Design review of the part built by this model. Coordinates are the model's own, in mm. Face numbers are marked on the shaded views. A direction names the side the tool comes from. Coordinates: 2 decimals unless noted, no trailing zeros. Loops run counter-clockwise (first coordinate to the right, second up) from the corner with the lowest first, then second, coordinate; pieces in that order, holes last. Notation, with made-up numbers: (33, 72.5) -> (76, 72.5) arc R28 cw to (76, 93.5) -> close; hole circle Ø9 at (51, 50.25). An arc over 180 degrees is marked (long way). Use a Markdown table: item, result. Add a question column.
Q1. Take a section at D-D on x = 10.5. Write out the cut boundary in (y, z) (3 decimals).
Q2. Draft analysis for pull direction Z (two halves, no side actions). For the marked faces 1, 2 and 3, state which applies: pulls with the +Z half, pulls with the -Z half, needs draft (parallel to the pull), parting line crosses it, or undercut.
Q3. For the marked faces 4, 5, 6, 7 and 8, list the 3-axis set-ups (+Z, -Z, +X, -X, +Y, -Y) from which the entire face can be reached by the end or side of a thin tool; tool diameter is ignored.
Q4. Clearance check with flat-ended pins moving along their axes: pin 1 Ø4 at (y, z) = (-14, 6.5) entering from +X; pin 2 Ø1.5 at (x, z) = (-22, 0) entering from -Y; pin 3 Ø5.5 at (x, z) = (10, -1.75) entering from -Y; pin 4 Ø4 at (x, y) = (13.5, -17.5) entering from -Z. State where each tip first meets the part, or that it passes through.
Q5. Take a section at A-A on y = 0. Write out the cut boundary in (x, z), plus the area to 3 significant figures.
Q6. Take a section at C-C on y = -14. Write out the cut boundary in (x, z), plus the area to 3 significant figures.
Q7. Take a section at B-B on x = -10. Write out the cut boundary in (y, z) (3 decimals).
Q8. For probe 1 along X at (y, z) = (-21, 10.5); probe 2 along X at (y, z) = (17.5, 8.5); probe 3 along X at (y, z) = (-3, 7.75), list the stretches that pass through material, from the lowest coordinate up.
Solid Edge part; units mm, degrees
sketch "Sketch1" plane through (0, 0, 0) normal (0, 0, 1) x (1, 0, 0)
  line L0 (23.5, -23.5) -> (20.5, -23.5)
  line L1 (20.5, 17) -> (20.5, -23.5)
  line L2 (-20.5, 17) -> (20.5, 17)
  line L3 (-20.5, -23.5) -> (-20.5, 17)
  line L4 (-20.5, -23.5) -> (-23.5, -23.5)
  line L5 (-23.5, -23.5) -> (-23.5, 23.5)
  line L6 (-23.5, 23.5) -> (23.5, 23.5)
  line L7 (23.5, 23.5) -> (23.5, -23.5)
  dimension "D1" = 20.5
  dimension "D2" = 20.5
  dimension "D3" = 23.5
  dimension "D4" = 20.5
  dimension "D5" = 23.5
extrude "ProtrusiónExtruida_1" add sketch "Sketch1" along normal mid plane 16
sketch "Sketch2" plane through (0, 0, 8) normal (0, 0, 1) x (1, 0, 0)
  line L0 (23.5, -23.5) -> (-23.5, -23.5)
  line L1 (-23.5, -23.5) -> (-23.5, 23.5)
  line L2 (-23.5, 23.5) -> (23.5, 23.5)
  line L3 (23.5, 23.5) -> (23.5, -23.5)
extrude "Protrusion1" add sketch "Sketch2" along normal blind 4
sketch "Sketch3" plane through (-23.5, 0, -2.5) normal (-1, 0, 0) x (0, 1, 0)
  line L0 (14, -4.5) -> (9, -4.5)
  line L1 (14, 0.5) -> (14, -4.5)
  dimension "D1" = 14
extrude "Cutout1" cut sketch "Sketch3" against normal through all material side at (-23.5, 11.5, 1.95)
sketch "Sketch4" plane through (0, 17, 0) normal (0, -1, 0) x (-1, 0, 0)
  line L0 (8.3401, 4.625) -> (11.6599, 4.625)
  line L1 (11.6599, 4.625) -> (13.3198, 1.75)
  line L2 (13.3198, 1.75) -> (11.6599, -1.125)
  line L3 (11.6599, -1.125) -> (8.3401, -1.125)
  line L4 (8.3401, -1.125) -> (6.6802, 1.75)
  line L5 (6.6802, 1.75) -> (8.3401, 4.625)
extrude "VaciadoExtruido_18" cut sketch "Sketch4" against normal blind 5
sketch "Sketch5" plane through (0, 23.5, -2.5) normal (0, 1, 0) x (1, 0, 0)
  circle A0 centre (-10, -0.75) radius 1.65
  dimension "D1" = 10
extrude "Cutout2" cut sketch "Sketch5" against normal up to next
chamfer "Chaflán_1" distance 10 angle 45 2 edges at (-23.5, 18.75, -8) (23.5, 18.75, -8)
fillet "Redondeo_5" radius 10 2 edges at (-13.5, 20.25, -8) (13.5, 20.25, -8)
sketch "Sketch6" plane through (0, -4.5, 8) normal (0, 0, -1) x (-1, 0, 0)
  line L0 (-22.7321, -13.5) -> (-19.2679, -13.5)
  line L1 (-19.2679, -13.5) -> (-17.5359, -16.5)
  line L2 (-17.5359, -16.5) -> (-19.2679, -19.5)
  line L3 (-19.2679, -19.5) -> (-22.7321, -19.5)
  line L4 (-24.8409, -19.8273) -> (-22.7321, -19.5)
  line L5 (-24.4641, -16.5) -> (-24.8409, -19.8273)
  line L6 (-24.4641, -16.5) -> (-22.7321, -13.5)
  line L7 (19.2679, -13.5) -> (22.7321, -13.5)
  line L8 (22.7321, -13.5) -> (24.4641, -16.5)
  line L9 (25.4467, -19.5) -> (24.4641, -16.5)
  line L10 (22.7321, -19.5) -> (25.4467, -19.5)
  line L11 (22.7321, -19.5) -> (19.2679, -19.5)
  line L12 (19.2679, -19.5) -> (17.5359, -16.5)
  line L13 (17.5359, -16.5) -> (19.2679, -13.5)
  line L14 (19.2679, 28.5) -> (22.7321, 28.5)
  line L15 (22.7321, 28.5) -> (25.2223, 28.8412)
  line L16 (25.2223, 28.8412) -> (24.4641, 25.5)
  line L17 (24.4641, 25.5) -> (22.7321, 22.5)
  line L18 (22.7321, 22.5) -> (19.2679, 22.5)
  line L19 (19.2679, 22.5) -> (17.5359, 25.5)
  line L20 (17.5359, 25.5) -> (15.8038, 28.5)
  line L21 (15.8038, 28.5) -> (19.2679, 28.5)
  line L22 (-22.7321, 28.5) -> (-19.2679, 28.5)
  line L23 (-19.2679, 28.5) -> (-15.8038, 28.5)
  line L24 (-15.8038, 28.5) -> (-17.5359, 25.5)
  line L25 (-17.5359, 25.5) -> (-19.2679, 22.5)
  line L26 (-19.2679, 22.5) -> (-22.7321, 22.5)
  line L27 (-22.7321, 22.5) -> (-24.4641, 25.5)
  line L28 (-25.1936, 28.5) -> (-24.4641, 25.5)
  line L29 (-22.7321, 28.5) -> (-25.1936, 28.5)
extrude "VaciadoExtruido_32" cut sketch "Sketch6" against normal blind 1 and the other way up to next
sketch "Sketch7" plane through (9, -9, 12) normal (0, 0, 1) x (0, -1, 0)
  circle A0 centre (-30, -30) radius 1.65
  circle A1 centre (12, -30) radius 1.65
  circle A2 centre (12, 12) radius 1.65
  circle A3 centre (-30, 12) radius 1.65
extrude "Cutout3" cut sketch "Sketch7" against normal up to next
sketch "Sketch8" plane through (0, -4.5, 8) normal (0, 0, -1) x (-1, 0, 0)
  line L0 (-2.75, -19) -> (2.75, -19)
  line L1 (2.75, -19) -> (2.75, -20.75)
  line L2 (2.75, -20.75) -> (-2.75, -20.75)
  line L3 (-2.75, -20.75) -> (-2.75, -19)
  dimension "D1" = 2.75
  dimension "D2" = 2.75
revolve "VaciadoPorRevolución_1" cut sketch "Sketch8" angle 90 about axis through (4.4935, -21.7, 8) along (-1, 0, 0)
sketch "Sketch9" plane through (0, -21.7, 11.25) normal (0, -1, 0) x (-1, 0, 0)
  line L0 (-2.75, 1.45) -> (2.75, 1.45)
  line L1 (2.75, 1.45) -> (2.75, -0.3)
  line L2 (2.75, -0.3) -> (-2.75, -0.3)
  line L3 (-2.75, -0.3) -> (-2.75, 1.45)
extrude "VaciadoExtruido_34" cut sketch "Sketch9" against normal blind 34
sketch "Sketch10" plane through (0, 12.3, 11.25) normal (0, -1, 0) x (-1, 0, 0)
  line L0 (-2.75, -0.3) -> (-2.75, 1.45)
  line L1 (-2.75, 1.45) -> (2.75, 1.45)
  line L2 (2.75, 1.45) -> (2.75, -0.3)
  line L3 (2.75, -0.3) -> (-2.75, -0.3)
revolve "RevolvedCutout1" cut sketch "Sketch10" angle 90 about axis through (2.8162, 12.3, 2.8) along (-1, 0, 0)
sketch "Sketch11" plane through (0, 18.25, 2.8) normal (0, 0, 1) x (1, 0, 0)
  line L0 (2.75, 1.05) -> (-2.75, 1.05)
  line L1 (-2.75, 1.05) -> (-2.75, 2.8)
  line L2 (-2.75, 2.8) -> (2.75, 2.8)
  line L3 (2.75, 2.8) -> (2.75, 1.05)
extrude "Cutout4" cut sketch "Sketch11" against normal up to next
fillet "Redondeo_6" radius 2 1 edges at (0, 19.3, -8)
sketch "Sketch12" plane through (22, -2, -8) normal (0, 0, -1) x (0, -1, 0)
  line L0 (-4.75, 0.25) -> (0.75, 0.25)
  line L1 (0.75, 0.25) -> (0.75, -1.5)
  line L2 (0.75, -1.5) -> (-4.75, -1.5)
  line L3 (-4.75, -1.5) -> (-4.75, 0.25)
  dimension "D1" = 4.75
  dimension "D2" = 0.75
extrude "Cutout5" cut sketch "Sketch12" against normal up to surface (16 mm away)
sketch "Sketch13" plane through (22.75, 0, 8) normal (0, 0, -1) x (-1, 0, 0)
  line L0 (1, 2.75) -> (-0.75, 2.75)
  line L1 (-0.75, 2.75) -> (-0.75, -2.75)
  line L2 (-0.75, -2.75) -> (1, -2.75)
  line L3 (1, -2.75) -> (1, 2.75)
revolve "VaciadoPorRevolución_3" cut sketch "Sketch13" angle 90 about axis through (20.25, 2.6731, 8) along (0, -1, 0)
sketch "Sketch14" plane through (20.25, 0, 11.25) normal (1, 0, 0) x (0, -1, 0)
  line L0 (-2.75, 1.75) -> (-2.75, 0)
  line L1 (-2.75, 0) -> (2.75, 0)
  line L2 (2.75, 0) -> (2.75, 1.75)
  line L3 (2.75, 1.75) -> (-2.75, 1.75)
extrude "VaciadoExtruido_37" cut sketch "Sketch14" against normal blind 33
mirror "Mirror1" about plane through (0, 0, 0) normal (1, 0, 0) of "Cutout2", "VaciadoExtruido_18", "Cutout5", "VaciadoPorRevolución_3", "VaciadoExtruido_37"
sketch "Sketch15" plane through (0, -4.5, 8) normal (0, 0, -1) x (0, -1, 0)
  line L0 (5, 27.5098) -> (5, -27.4354)
extrude "Cutout10" cut sketch "Sketch15" along normal through all material side at (-0.0372, -9.55, 8)
sketch "Sketch16" plane through (0, -4, 11.25) normal (0, 0, -1) x (-1, 0, 0)
  line L0 (-2.75, 1.25) -> (-2.75, -2.5)
  line L1 (-2.75, -2.5) -> (2.75, -2.5)
  line L2 (2.75, 1.25) -> (2.75, -2.5)
  line L3 (6.5, 1.25) -> (2.75, 1.25)
  line L4 (6.5, 1.25) -> (6.5, 6.75)
  line L5 (6.5, 6.75) -> (2.75, 6.75)
  line L6 (2.75, 10.5) -> (2.75, 6.75)
  line L7 (2.75, 10.5) -> (-2.75, 10.5)
  line L8 (-2.75, 10.5) -> (-2.75, 6.75)
  line L9 (-2.75, 6.75) -> (-6.5, 6.75)
  line L10 (-6.5, 6.75) -> (-6.5, 1.25)
  line L11 (-2.75, 1.25) -> (-6.5, 1.25)
extrude "Cutout11" cut sketch "Sketch16" against normal up to next
sketch "Sketch17" plane through (0, -3.25, 8) normal (0, 0, -1) x (1, 0, 0)
  line L0 (-2.75, 16.75) -> (2.75, 16.75)
  line L1 (2.75, 16.75) -> (2.75, 20.25)
  line L2 (2.75, 20.25) -> (-2.75, 20.25)
  line L3 (-2.75, 16.75) -> (-2.75, 20.25)
extrude "Cutout12" cut sketch "Sketch17" against normal up to next
properties material "Abs 15"
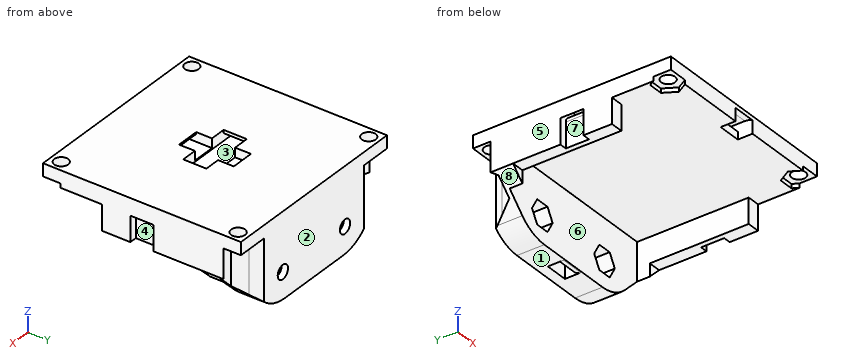
Answer list:
| question | item | result |
|---|---|---|
| 1 | outline | (-23.5, 8) -> (17, 8) -> (17, 1.125) -> (22, 1.125) -> (22, -0.178) -> (23.5, -0.178) -> (23.5, 12) -> (-23.5, 12) -> close; (17, -7.935) -> (23.5, -7.935) -> (23.5, -3.322) -> (22, -3.322) -> (22, -4.625) -> (17, -4.625) -> close; hole (-2.75, 9.5) -> (2.75, 9.5) -> (2.75, 11.25) -> (-2.75, 11.25) -> close |
| 2 | face 1 | pulls with the -Z half |
| 2 | face 2 | needs draft |
| 2 | face 3 | undercut |
| 3 | face 4 | -Z, +X |
| 3 | face 5 | +Z, -Z, -X, +Y, -Y |
| 3 | face 6 | -Z, -Y |
| 3 | face 7 | -Z, -X |
| 3 | face 8 | -Z, -X, +Y, -Y |
| 4 | pin 1 | x = 23.5 |
| 4 | pin 2 | y = 14 |
| 4 | pin 3 | y = 22 |
| 4 | pin 4 | z = 8 |
| 5 | outline | (-23.5, 8) arc R3.25 cw to (-20.25, 11.25) -> (-6.5, 11.25) -> (-6.5, 12) -> (-23.5, 12) -> close; (-21.75, 2) -> (-20.5, 2) -> (-20.5, 8) -> (20.5, 8) -> (20.5, 2) -> (21.75, 2) -> (21.75, 8) arc R1.5 ccw to (20.25, 9.5) -> (-20.25, 9.5) arc R1.5 ccw to (-21.75, 8) -> close; (6.5, 11.25) -> (20.25, 11.25) arc R3.25 cw to (23.5, 8) -> (23.5, 12) -> (6.5, 12) -> close |
| 5 | area | 109 mm² |
| 6 | outline | (-23.5, 8) -> (23.5, 8) -> (23.5, 12) -> (-23.5, 12) -> close; hole (-2.75, 9.8) -> (2.75, 9.8) -> (2.75, 11.55) -> (-2.75, 11.55) -> close |
| 6 | area | 178 mm² |
| 7 | outline | (-23.5, 8) -> (17, 8) -> (17, 1.125) -> (22, 1.125) -> (22, -0.1) -> (23.5, -0.1) -> (23.5, 12) -> (-23.5, 12) -> close; (17, -7.979) -> (23.5, -7.979) -> (23.5, -3.4) -> (22, -3.4) -> (22, -4.625) -> (17, -4.625) -> close; hole (-2.75, 9.5) -> (2.75, 9.5) -> (2.75, 11.25) -> (-2.75, 11.25) -> close |
| 8 | probe 1 | -23.5 to -22.65, -19.35 to -2.75, 2.75 to 19.35, 22.65 to 23.5 |
| 8 | probe 2 | -23.5 to -2.75, 2.75 to 23.5 |
| 8 | probe 3 | -23.5 to -20.5, 20.5 to 23.5 |
